Input: part model. Units: mm. Frame: model coordinates. Face numbers are marked on the shaded views. A direction names the side the tool comes from. Round coordinates to 2 decimals unless told otherwise and drop trailing zeros. Loops run counter-clockwise (first coordinate to the right, second up) from the corner with the lowest first, then second, coordinate; pieces in that order, holes last. Notation, with made-up numbers: (3, 59) -> (56, 59) arc R9 ccw to (56, 76) -> close; hole circle Ø7 at (38, 38.5). An arc over 180 degrees is marked (long way). Answer in a Markdown table with one row per item. Add a question column.
Q1. Section D-D, the plane y = 0. Give the number of separate pieces and of enclosed holes in the cut face, and give its area (3 significant figures).
Q2. Reachability of the marked faces 1, 2, 3 and 4 from +Z, -Z, +X, -X, +Y, -Y: full face, straight path, thin tool, end or side. Return the list, or none.
Q3. Section C-C, the plane x = -20.5. Output: boundary loops of the cut face in (y, z), and give its area (3 significant figures).
Q4. Pin query (flat end, axial travel): pin 1 (2.5 mm diameter, centred on x = -5.7, y = 0, fed in from +Z); pin 2 (7 mm diameter, centred on x = 10.5, z = 4, fed in from +Y); pin 3 (2 mm diameter, centred on y = -7.5, z = 5.5, fed in from -X); pin 4 (8 mm diameter, centred on x = -14.5, z = 11, fed in from +Y). Return the tip coordinate at first contact, or that it passes through.
Q5. Section B-B, the plane x = -5.7. Output: boundary loops of the cut face in (y, z).
Q6. Ray query, L1, parallel to X at y = -3.5, z = 7; L2, parallel to X at y = 5, z = 3.5; L3, parallel to Y at x = 5.7, z = 15.25. Return the intervals inside material, ascending. Write a range as from..to.
Q7. Section A-A, the plane x = 17. Output: boundary loops of the cut face in (y, z), and give its area (3 significant figures).
```python
from build123d import *

# Parameters (mm, degrees)
F0_W      = 84.5
F0_H      = 12
F1_DEPTH  = 20
F3_DEPTH  = 3
F4_DEPTH  = 25
F5_R      = 1.6
F5_W      = 6
F5_H      = 11.54
F5_R_2    = 2
F6_DEPTH  = 5
F7_DEPTH  = 25
F8_R      = 2
F8_R_2    = 1.6
F9_DEPTH  = 10
F10_R     = 1.6
F11_DEPTH = 25
F12_R     = 1.6
F13_DEPTH = 12
F14_DEPTH = 10


# Not quite as in the source:
# - a pattern or mirror of a feature is missing from the dataset's text; its kind, count and spacing are read off the source's solid


with BuildPart() as f1:
    # F0 (on Top) → F1 (new body)
    with BuildSketch(Plane.XY):
        Rectangle(F0_W, F0_H)
    extrude(amount=F1_DEPTH)

    # F2 (on face) → F3 (cut)
    with BuildSketch(Plane(origin=(0, 6, 0), x_dir=(-1, 0, 0), z_dir=(0, 1, 0))):
        with BuildLine():
            ThreePointArc((11, 8), (17, 2), (23, 8))
            ThreePointArc((23, 8), (17, 14), (11, 8))
        make_face()
        with BuildLine():
            Line((23, 2.7084973779), (23, 8))
            ThreePointArc((23, 8), (17, 2), (11, 8))
            Line((11, 8), (11, 2.7084973779))
            ThreePointArc((11, 2.7084973779), (13.7084973779, 0.7084973779), (17, 0))
            ThreePointArc((17, 0), (20.2915026221, 0.7084973779), (23, 2.7084973779))
        make_face()
        with BuildLine():
            Line((23, 0), (23, 2.7084973779))
            ThreePointArc((23, 2.7084973779), (20.2915026221, 0.7084973779), (17, 0))
            Line((17, 0), (23, 0))
        make_face()
        with BuildLine():
            ThreePointArc((25, 8), (24.4833147735, 5.1715728753), (23, 2.7084973779))
            Line((23, 2.7084973779), (23, 0))
            Line((23, 0), (25, 0))
            Line((25, 0), (25, 8))
        make_face()
        with BuildLine():
            ThreePointArc((17, 0), (13.7084973779, 0.7084973779), (11, 2.7084973779))
            Line((11, 2.7084973779), (11, 0))
            Line((11, 0), (17, 0))
        make_face()
        with BuildLine():
            Line((11, 0), (11, 2.7084973779))
            ThreePointArc((11, 2.7084973779), (9.5166852265, 5.1715728753), (9, 8))
            Line((9, 8), (9, 0))
            Line((9, 0), (11, 0))
        make_face()
        with BuildLine():
            ThreePointArc((11, 8), (17, 14), (23, 8))
            Line((23, 8), (23, 2.7084973779))
            ThreePointArc((23, 2.7084973779), (24.4833147735, 5.1715728753), (25, 8))
            ThreePointArc((25, 8), (17, 16), (9, 8))
            ThreePointArc((9, 8), (9.5166852265, 5.1715728753), (11, 2.7084973779))
            Line((11, 2.7084973779), (11, 8))
        make_face()
    f3 = extrude(amount=-F3_DEPTH, mode=Mode.SUBTRACT)

    # F3_copies: F3 across plane
    add(f3.mirror(Plane(origin=(0, 0, 0), x_dir=(0, 0, -1), z_dir=(0, -1, 0))), mode=Mode.SUBTRACT)

    # F2 (on face) → F4 (cut)
    with BuildSketch(Plane(origin=(0, 6, 0), x_dir=(-1, 0, 0), z_dir=(0, 1, 0))):
        with BuildLine():
            Line((23, 2.7084973779), (23, 8))
            ThreePointArc((23, 8), (17, 2), (11, 8))
            Line((11, 8), (11, 2.7084973779))
            ThreePointArc((11, 2.7084973779), (13.7084973779, 0.7084973779), (17, 0))
            ThreePointArc((17, 0), (20.2915026221, 0.7084973779), (23, 2.7084973779))
        make_face()
        with BuildLine():
            Line((23, 0), (23, 2.7084973779))
            ThreePointArc((23, 2.7084973779), (20.2915026221, 0.7084973779), (17, 0))
            Line((17, 0), (23, 0))
        make_face()
        with BuildLine():
            ThreePointArc((17, 0), (13.7084973779, 0.7084973779), (11, 2.7084973779))
            Line((11, 2.7084973779), (11, 0))
            Line((11, 0), (17, 0))
        make_face()
        with BuildLine():
            ThreePointArc((11, 8), (17, 2), (23, 8))
            ThreePointArc((23, 8), (17, 14), (11, 8))
        make_face()
    extrude(amount=-F4_DEPTH, mode=Mode.SUBTRACT)

    # F5 (on face) → F6 (join)
    with BuildSketch(Plane.XZ.offset(6)):
        with BuildLine():
            ThreePointArc((12, 8), (10.430589025, 11.1768281338), (6.9538815041, 11.8607817981))
            ThreePointArc((6.9538815041, 11.8607817981), (4, 8), (6.9538815041, 4.1392182019))
            ThreePointArc((6.9538815041, 4.1392182019), (10.430589025, 4.8231718662), (12, 8))
        make_face()
        with Locations((8, 8)):
            Circle(F5_R, mode=Mode.SUBTRACT)
        with BuildLine():
            Line((14, 2.23), (14, 13.77))
            Line((14, 13.77), (6.9538815041, 11.8607817981))
            ThreePointArc((6.9538815041, 11.8607817981), (10.430589025, 11.1768281338), (12, 8))
            ThreePointArc((12, 8), (10.430589025, 4.8231718662), (6.9538815041, 4.1392182019))
            Line((6.9538815041, 4.1392182019), (14, 2.23))
        make_face()
        with Locations((17, 8)):
            Rectangle(F5_W, F5_H)
        with Locations((17, 8)):
            Circle(F5_R_2, mode=Mode.SUBTRACT)
        with BuildLine():
            Line((27.0461184959, 11.8607817981), (20, 13.77))
            Line((20, 13.77), (20, 2.23))
            Line((20, 2.23), (27.0461184959, 4.1392182019))
            ThreePointArc((27.0461184959, 4.1392182019), (22, 8), (27.0461184959, 11.8607817981))
        make_face()
        with BuildLine():
            ThreePointArc((30, 8), (29.1768281338, 10.430589025), (27.0461184959, 11.8607817981))
            ThreePointArc((27.0461184959, 11.8607817981), (22, 8), (27.0461184959, 4.1392182019))
            ThreePointArc((27.0461184959, 4.1392182019), (29.1768281338, 5.569410975), (30, 8))
        make_face()
        with Locations((26, 8)):
            Circle(F5_R, mode=Mode.SUBTRACT)
    extrude(amount=F6_DEPTH)

    # F5 (on face) → F7 (cut)
    with BuildSketch(Plane.XZ.offset(6)):
        with Locations((8, 8)):
            Circle(F5_R)
        with Locations((17, 8)):
            Circle(F5_R_2)
        with Locations((26, 8)):
            Circle(F5_R)
    extrude(amount=-F7_DEPTH, mode=Mode.SUBTRACT)

    # F8 (on face) → F9 (cut)
    with BuildSketch(Plane(origin=(0, 6, 0), x_dir=(-1, 0, 0), z_dir=(0, 1, 0))):
        with BuildLine():
            Line((-6.9538815041, 11.8607817981), (-14, 13.77))
            Line((-14, 13.77), (-20, 13.77))
            Line((-20, 13.77), (-27.0461184959, 11.8607817981))
            ThreePointArc((-27.0461184959, 11.8607817981), (-23.569410975, 11.1768281338), (-22, 8))
            ThreePointArc((-22, 8), (-23.569410975, 4.8231718662), (-27.0461184959, 4.1392182019))
            Line((-27.0461184959, 4.1392182019), (-20, 2.23))
            Line((-20, 2.23), (-14, 2.23))
            Line((-14, 2.23), (-6.9538815041, 4.1392182019))
            ThreePointArc((-6.9538815041, 4.1392182019), (-12, 8), (-6.9538815041, 11.8607817981))
        make_face()
        with Locations((-17, 8)):
            Circle(F8_R, mode=Mode.SUBTRACT)
        with BuildLine():
            ThreePointArc((-4, 8), (-4.8231718662, 10.430589025), (-6.9538815041, 11.8607817981))
            ThreePointArc((-6.9538815041, 11.8607817981), (-12, 8), (-6.9538815041, 4.1392182019))
            ThreePointArc((-6.9538815041, 4.1392182019), (-4.8231718662, 5.569410975), (-4, 8))
        make_face()
        with Locations((-8, 8)):
            Circle(F8_R_2, mode=Mode.SUBTRACT)
        with BuildLine():
            ThreePointArc((-22, 8), (-23.569410975, 11.1768281338), (-27.0461184959, 11.8607817981))
            ThreePointArc((-27.0461184959, 11.8607817981), (-29.1768281338, 10.430589025), (-30, 8))
            ThreePointArc((-30, 8), (-29.1768281338, 5.569410975), (-27.0461184959, 4.1392182019))
            ThreePointArc((-27.0461184959, 4.1392182019), (-23.569410975, 4.8231718662), (-22, 8))
        make_face()
        with Locations((-26, 8)):
            Circle(F8_R_2, mode=Mode.SUBTRACT)
    extrude(amount=-F9_DEPTH, mode=Mode.SUBTRACT)

    # F10 (on face) → F11 (cut)
    with BuildSketch(Plane.XY.offset(20)):
        with Locations((-36.7, 0)):
            Circle(F10_R)
        with Locations((-5.7, 0)):
            Circle(F10_R)
        with Locations((5.7, 0)):
            Circle(F10_R)
        with Locations((36.7, 0)):
            Circle(F10_R)
    extrude(amount=-F11_DEPTH, mode=Mode.SUBTRACT)

    # F12 (on face) → F13 (cut)
    with BuildSketch(Plane(origin=(0, 6, 0), x_dir=(-1, 0, 0), z_dir=(0, 1, 0))):
        Polygon((-6.5680812925, 10.4061605963), (-9.3678368482, 10.443158275), (-10.7997555557, 8.0369976787), (-9.4319187075, 5.5938394037), (-6.6321631518, 5.556841725), (-5.2002444443, 7.9630023213), align=None)
        with Locations((-8, 8)):
            Circle(F12_R, mode=Mode.SUBTRACT)
        Polygon((-28.7997555557, 7.9630023213), (-27.3678368482, 5.556841725), (-24.5680812925, 5.5938394037), (-23.2002444443, 8.0369976787), (-24.6321631518, 10.443158275), (-27.4319187075, 10.4061605963), align=None)
        with Locations((-26, 8)):
            Circle(F12_R, mode=Mode.SUBTRACT)
    extrude(amount=-F13_DEPTH, mode=Mode.SUBTRACT)

    # F8 (on face) → F14 (cut)
    with BuildSketch(Plane(origin=(0, 6, 0), x_dir=(-1, 0, 0), z_dir=(0, 1, 0))):
        with BuildLine():
            ThreePointArc((-8.3944853395, 0), (-7.0789353021, 1.8624403356), (-6.9538815041, 4.1392182019))
            Line((-6.9538815041, 4.1392182019), (-14, 2.23))
            Line((-14, 2.23), (-20, 2.23))
            Line((-20, 2.23), (-27.0461184959, 4.1392182019))
            ThreePointArc((-27.0461184959, 4.1392182019), (-29.1768281338, 5.569410975), (-30, 8))
            Line((-30, 8), (-30, 0))
            Line((-30, 0), (-8.3944853395, 0))
        make_face()
    extrude(amount=-F14_DEPTH, mode=Mode.SUBTRACT)


solid = f1.part
```
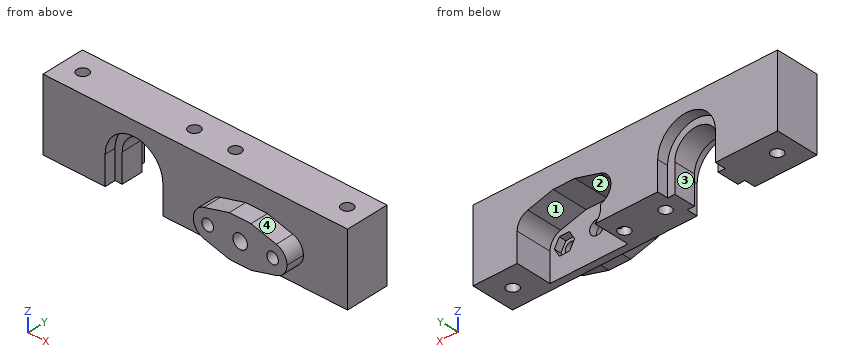
Answer block:
| question | item | result |
|---|---|---|
| 1 | separate pieces | 6 |
| 1 | enclosed holes | 0 |
| 1 | area | 991 mm^2 |
| 2 | face 1 | -Z, +Y |
| 2 | face 2 | +Y |
| 2 | face 3 | -Z, +Y, -Y |
| 2 | face 4 | +Z, +X, -Y |
| 3 | outline | (-6, 15.19) -> (-3, 15.19) -> (-3, 12.87) -> (3, 12.87) -> (3, 15.19) -> (6, 15.19) -> (6, 20) -> (-6, 20) -> close |
| 3 | area | 71.6 mm^2 |
| 4 | pin 1 | through |
| 4 | pin 2 | y = -4 |
| 4 | pin 3 | x = 4.29 |
| 4 | pin 4 | y = 3 |
| 5 | outline | (-6, 0) -> (-1.6, 0) -> (-1.6, 20) -> (-6, 20) -> close; (1.6, 0) -> (6, 0) -> (6, 20) -> (1.6, 20) -> close |
| 6 | L1 | -42.25..-25, -9..4.13, 30..42.25 |
| 6 | L2 | -42.25..-25, -9..6.86, 30..42.25 |
| 6 | L3 | -6..-1.6, 1.6..6 |
| 7 | outline | (-11, 2.23) -> (-6, 2.23) -> (-6, 0) -> (-4, 0) -> (-4, 6) -> (-11, 6) -> close; (-11, 10) -> (-4, 10) -> (-4, 13.77) -> (6, 13.77) -> (6, 20) -> (-6, 20) -> (-6, 13.77) -> (-11, 13.77) -> close |
| 7 | area | 132 mm^2 |
